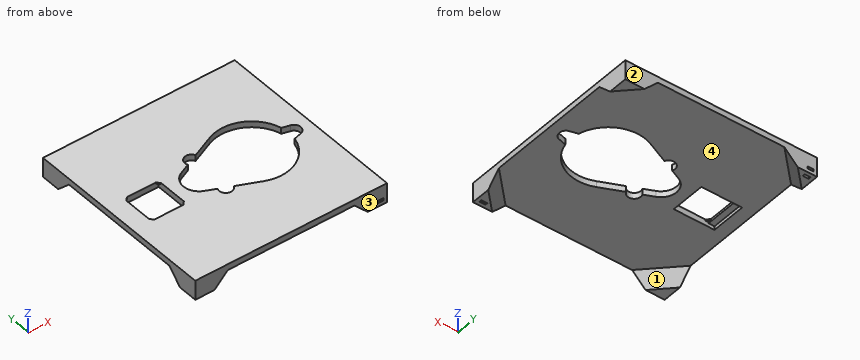
from build123d import *

# Parameters (mm, degrees)
SKETCH1_W           = 160
SKETCH1_H           = 160
SKETCH1_W_2         = 29
SKETCH1_H_2         = 29
BOSS_EXTRUDE1_DEPTH = 5
BOSS_EXTRUDE2_DEPTH = 1
SKETCH5_W           = 5
SKETCH5_H           = 29
CUT_EXTRUDE2_DEPTH  = 3
BOSS_EXTRUDE3_DEPTH = 11.22
BOSS_EXTRUDE5_DEPTH = 6.47787
BOSS_EXTRUDE6_DEPTH = 6.47787
BOSS_EXTRUDE7_DEPTH = 6.47787
BOSS_EXTRUDE8_DEPTH = 6.47787
SKETCH16_W          = 180
SKETCH16_H          = 180
SKETCH16_W_2        = 160
SKETCH16_H_2        = 160
CUT_EXTRUDE3_DEPTH  = 47
SKETCH18_W          = 5
SKETCH18_H          = 2
SKETCH19_W          = 5
SKETCH19_H          = 2


with BuildPart() as part:
    # Sketch1 → Boss-Extrude1 (new body)
    with BuildSketch(Plane(origin=(0, 0, 0), x_dir=(0, 1, 0), z_dir=(0, 0, 1))):
        with Locations((80, 80)):
            Rectangle(SKETCH1_W, SKETCH1_H)
        with BuildLine():
            Line((68.137582786, 98.618181818), (64.387982104, 90.254547554))
            ThreePointArc((64.387982104, 90.254547554), (56.981285025, 87.55), (59.88970449, 80.220959455))
            Line((59.88970449, 80.220959455), (51.712697414, 61.981818182))
            ThreePointArc((51.712697414, 61.981818182), (52.218398749, 35.545632261), (72.935219616, 19.115751158))
            Line((72.935219616, 19.115751158), (74.687407955, 12.576495252))
            ThreePointArc((74.687407955, 12.576495252), (80, 8.5), (85.312592045, 12.576495252))
            Line((85.312592045, 12.576495252), (87.064780384, 19.115751158))
            ThreePointArc((87.064780384, 19.115751158), (107.781601251, 35.545632261), (108.287302586, 61.981818182))
            Line((108.287302586, 61.981818182), (100.11029551, 80.220959455))
            ThreePointArc((100.11029551, 80.220959455), (103.018714975, 87.55), (95.612017896, 90.254547554))
            Line((95.612017896, 90.254547554), (91.862417214, 98.618181818))
            ThreePointArc((91.862417214, 98.618181818), (80, 106.3), (68.137582786, 98.618181818))
        make_face(mode=Mode.SUBTRACT)
        with Locations((80, 130)):
            Rectangle(SKETCH1_W_2, SKETCH1_H_2, mode=Mode.SUBTRACT)
    extrude(amount=BOSS_EXTRUDE1_DEPTH)

    # Sketch3 → Boss-Extrude2 (add)
    with BuildSketch(Plane.XY.offset(5)):
        Polygon((-144.5, 92), (-142, 94.5), (-144.5, 94.5), align=None)
        Polygon((-144.5, 65.5), (-142, 65.5), (-144.5, 68), align=None)
        Polygon((-115.5, 65.5), (-118, 65.5), (-115.5, 68), align=None)
        Polygon((-115.5, 94.5), (-115.5, 92), (-118, 94.5), align=None)
    extrude(amount=-BOSS_EXTRUDE2_DEPTH)

    # Sketch5 → Cut-Extrude2 (cut)
    with BuildSketch(Plane(origin=(0, 0, 0), x_dir=(1, 0, 0), z_dir=(0, 0, -1))):
        with Locations((-147, -80)):
            Rectangle(SKETCH5_W, SKETCH5_H)
    extrude(amount=-CUT_EXTRUDE2_DEPTH, mode=Mode.SUBTRACT)

    # Sketch6 → Boss-Extrude3 (add)
    with BuildSketch(Plane(origin=(0, 0, 0), x_dir=(1, 0, 0), z_dir=(0, 0, -1))):
        Polygon((-160, -16), (-160, 0), (-144, 0), align=None)
        Polygon((-144, -160), (-160, -160), (-160, -144), align=None)
        Polygon((0, -160), (-16, -160), (0, -144), align=None)
        Polygon((0, 0), (-16, 0), (0, -16), align=None)
    extrude(amount=BOSS_EXTRUDE3_DEPTH)

    # Sketch12 → Boss-Extrude5 (add)
    with BuildSketch(Plane(origin=(44.26, 44.26, 44.26), x_dir=(0.8164965809277263, -0.40824829046386296, -0.4082482904638628), z_dir=(0.5773502691896256, 0.5773502691896261, 0.5773502691896258))):
        Polygon((-54.207208008, 93.889638406), (-87.544763407, 113.13708499), (-73.80312595, 121.070823075), (-54.207208008, 109.757114576), align=None)
    extrude(amount=BOSS_EXTRUDE5_DEPTH)

    # Sketch13 → Boss-Extrude6 (add)
    with BuildSketch(Plane(origin=(-97.593333333, 97.593333333, 97.593333333), x_dir=(0.4082482904638652, -0.4082482904638646, 0.8164965809277241), z_dir=(-0.577350269189624, 0.5773502691896251, 0.5773502691896285))):
        Polygon((-133.268571939, 11.313708499), (-119.526934482, 19.247446584), (-119.526934482, -19.247446584), (-133.268571939, -11.313708499), align=None)
    extrude(amount=BOSS_EXTRUDE6_DEPTH)

    # Sketch14 → Boss-Extrude7 (add)
    with BuildSketch(Plane(origin=(-44.26, -44.26, 44.26), x_dir=(0.40824829046386135, 0.40824829046386096, 0.8164965809277279), z_dir=(-0.5773502691896302, -0.5773502691896242, 0.5773502691896232))):
        Polygon((-54.207208008, 132.384531574), (-67.948845465, 124.450793489), (-67.948845465, 101.823376491), (-54.207208008, 93.889638406), align=None)
    extrude(amount=BOSS_EXTRUDE7_DEPTH)

    # Sketch15 → Boss-Extrude8 (add)
    with BuildSketch(Plane(origin=(-9.073333333, 9.073333333, -9.073333333), x_dir=(-0.8164965809277261, -0.40824829046386324, 0.40824829046386274), z_dir=(0.5773502691896257, -0.5773502691896257, 0.577350269189626))):
        Polygon((-11.112518466, -19.247446584), (22.225036933, 0), (8.483399476, 7.933738085), (-11.112518466, -3.379970414), align=None)
    extrude(amount=BOSS_EXTRUDE8_DEPTH)

    # Sketch16 → Cut-Extrude3 (cut)
    with BuildSketch(Plane.XY.offset(5)):
        with Locations((-80, 80)):
            Rectangle(SKETCH16_W, SKETCH16_H)
        with Locations((-80, 80)):
            Rectangle(SKETCH16_W_2, SKETCH16_H_2, mode=Mode.SUBTRACT)
    extrude(amount=-CUT_EXTRUDE3_DEPTH, mode=Mode.SUBTRACT)

    # Sketch18 → Cut-Revolve1 (revolve, cut)
    with BuildSketch(Plane(origin=(0, 0, -11.22), x_dir=(1, 0, 0), z_dir=(0, 0, -1))):
        with Locations((-5.5, -4)):
            Rectangle(SKETCH18_W, SKETCH18_H)
    revolve(axis=Axis((0, 0, -11.22), (-1, 0, 0)), mode=Mode.SUBTRACT)

    # Sketch19 → Cut-Revolve2 (revolve, cut)
    with BuildSketch(Plane(origin=(0, 0, -11.22), x_dir=(1, 0, 0), z_dir=(0, 0, -1))):
        with Locations((-154.5, -156)):
            Rectangle(SKETCH19_W, SKETCH19_H)
    revolve(axis=Axis((-160, 160, -11.22), (1, 0, 0)), mode=Mode.SUBTRACT)


solid = part.part
The listing builds one solid part. Answer for the finished solid, in the listing's coordinates (mm). Face numbers are marked on the shaded views. A direction names the side the tool comes from. Give positions to 0.01 mm unless a question says otherwise; leave off trailing zeros. Loops run counter-clockwise (first coordinate to the right, second up) from the corner with the lowest first, then second, coordinate; pieces in that order, holes last. Notation, with made-up numbers: (89, 41) - (131, 41) arc R22 cw to (131, 55) - close; hole circle Ø4 at (35, -25.75). An arc over 180 degrees is marked (long way). Answer as a JSON object with one key per item and string values.
1. Find the intervals of material crossed by L1, parallel to Y at x = -135.5, z = 3.75; L2, parallel to Z at x = -134.5, y = 148; L3, parallel to Y at x = -30, z = 3.5, in increasing order. Write a range as [from, to].
Determined:
{"L1": "[0, 65.5], [94.5, 160]", "L2": "[0, 5]", "L3": "[0, 55.74], [104.26, 160]"}
2. Flat-ended cylindrical pins translate along their axes: pin 1 Ø2 at (x, y) = (-117, 93) entering from -Z; pin 2 Ø5 at (y, z) = (41.5, -3.5) entering from +X; pin 3 Ø1 at (x, y) = (-100.5, 55) entering from -Z; pin 4 Ø2.5 at (x, y) = (-148, 85.5) entering from -Z. Find the tip coordinate at first contact, or state that the pin passes through.
Determined:
{"pin 1": "z = 4", "pin 2": "through", "pin 3": "z = 0", "pin 4": "z = 3"}
3. For the marked faces 1 and 2, determine the directions among +Z, -Z, +X, -X, +Y, -Y from which every point of the face is accessible in a straight line to the end or side of a thin tool.
Determined:
{"face 1": "-Z", "face 2": "+Z, -Z, +X, -X, +Y"}
4. A cutting plane is placed at D-D (y = 19.5). Write down the section's boundary in (x, z).
Determined:
{"outline": "(-160, -7.72) - (-152.28, 0) - (-7.72, 0) - (0, -7.72) - (0, 5) - (-160, 5) - close"}
5. A cutting plane is placed at A-A (x = -129). Write down the section's boundary in (y, z), then the cut area to 3 significant figures.
Determined:
{"outline": "(0, 0) - (65.5, 0) - (65.5, 5) - (0, 5) - close; (94.5, 0) - (160, 0) - (160, 5) - (94.5, 5) - close", "area": "655 mm²"}
6. A cutting plane is placed at C-C (y = 98). Write down the section's boundary in (x, z), then the cut area to 3 significant figures.
Determined:
{"outline": "(-160, 0) - (-90.8, 0) - (-90.8, 5) - (-160, 5) - close; (-24.06, 0) - (0, 0) - (0, 5) - (-24.06, 5) - close", "area": "466 mm²"}
7. A cutting plane is placed at B-B (z = -2.5). Write down the section's boundary in (x, y).
Determined:
{"outline": "(-160, 0) - (-135.28, 0) - (-160, 24.72) - close; (-160, 135.28) - (-135.28, 160) - (-160, 160) - close; (-24.72, 0) - (0, 0) - (0, 24.72) - close; (-24.72, 160) - (0, 135.28) - (0, 160) - close"}
8. For a pull along X with two mould halves and no side action, classify the marked faces 3 and 4 as pulls with the +X half, pulls with the -X half, needs draft (parallel to the pull), parting line crosses it, or undercut.
Determined:
{"face 3": "needs draft", "face 4": "undercut"}
